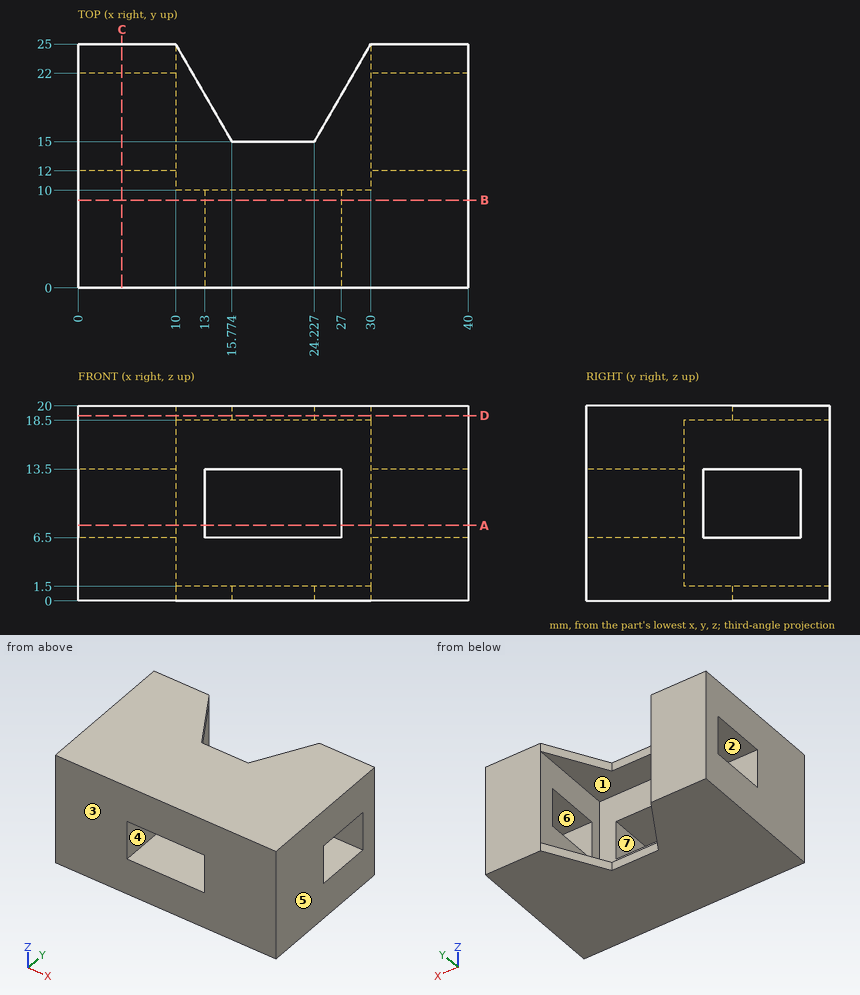
Input: dimensioned drawing with shaded views. Units: mm. Origin: part minimum x, y, z. A direction names the side the tool comes from. Give positions to 0.01 mm unless a question says otherwise; leave off trailing zeros. Write each loop counter-clockwise with the first axis right and the second up, starting at its lowest first coordinate (ties: lowest second). Pieces come first, ordered by that corner, then holes. Notation, with made-up numbers: (-15, -5) -> (21, -5) arc R11 cw to (21, 1) -> close; hole circle Ø3 at (27, -14.5). An arc over 180 degrees is marked (long way). Answer as a JSON object with one key per item and string values.
1. Access query for the marked faces 1, 2, 3 and 4. Directions: +Z, -Z, +X, -X, +Y, -Y. A direction counts if a zero-diameter tool reaches every point of the face in a straight line with its end or side. Return the directions, or none.
Ans:
{"face 1": "+Y", "face 2": "+X, -X", "face 3": "+Z, -Z, +X, -X, -Y", "face 4": "+Y, -Y"}
2. Cut plane B-B on y = 9. Output: boundary loops of the cut face in (x, z).
Ans:
{"outline": "(0, 0) -> (40, 0) -> (40, 20) -> (0, 20) -> close; hole (13, 6.5) -> (27, 6.5) -> (27, 13.5) -> (13, 13.5) -> close"}
3. Cut plane D-D on z = 19. Output: boundary loops of the cut face in (x, y).
Ans:
{"outline": "(0, 0) -> (40, 0) -> (40, 25) -> (30, 25) -> (24.23, 15) -> (15.77, 15) -> (10, 25) -> (0, 25) -> close"}
4. Contact query for a flat-ended pin moving along its axis: pin 1 (1 mm diameter, centred on x = 23, z = 12.5, fed in from +Y). Output: stop coordinate, or through.
Ans:
{"pin 1": "passes through"}
5. Cut plane C-C on x = 4.5. Output: boundary loops of the cut face in (y, z), and give its area (3 significant figures).
Ans:
{"outline": "(0, 0) -> (25, 0) -> (25, 20) -> (0, 20) -> close; hole (12, 6.5) -> (22, 6.5) -> (22, 13.5) -> (12, 13.5) -> close", "area": "430 mm^2"}
6. Ray query, probe 1 along X at (y, z) = (11.75, 17); probe 2 along Z at (x, y) = (33.5, 17.25); probe 3 along Y at (x, z) = (3, 8.5). Return the intervals inside material, ascending. Write a range as from..to.
Ans:
{"probe 1": "x = 0..10, 30..40", "probe 2": "z = 0..6.5, 13.5..20", "probe 3": "y = 0..12, 22..25"}
7. Cut plane A-A on z = 7.75. Output: boundary loops of the cut face in (x, y), and give its area (3 significant figures).
Ans:
{"outline": "(0, 0) -> (13, 0) -> (13, 10) -> (10, 10) -> (10, 12) -> (0, 12) -> close; (0, 22) -> (10, 22) -> (10, 25) -> (0, 25) -> close; (27, 0) -> (40, 0) -> (40, 12) -> (30, 12) -> (30, 10) -> (27, 10) -> close; (30, 22) -> (40, 22) -> (40, 25) -> (30, 25) -> close", "area": "360 mm^2"}
8. Mould query, pull axis X, two halves, no side actions, for the marked faces 5, 6 and 7. Classes: pulls with the +X half, pulls with the -X half, needs draft (parallel to the pull), parting line crosses it, or undercut.
Ans:
{"face 5": "pulls with the +X half", "face 6": "needs draft", "face 7": "undercut"}
